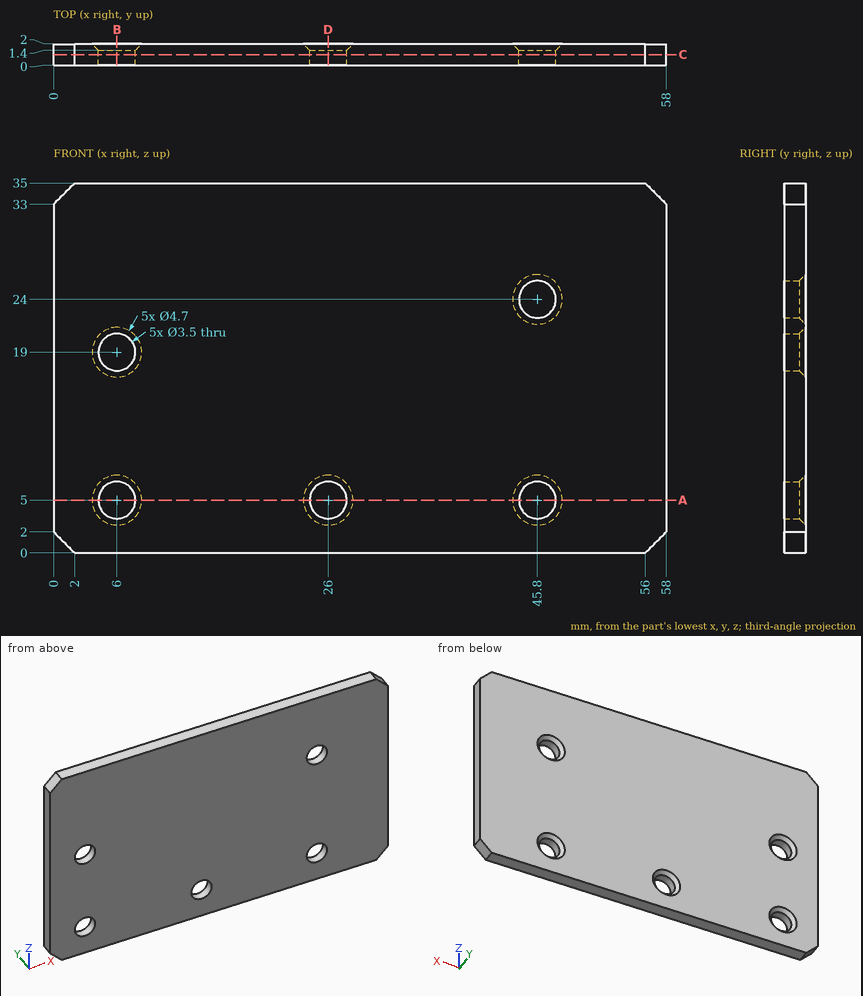
Drawing for the job (mm, zero at the part's lowest x, y, z). Give positions to 0.01 mm unless a question says otherwise; leave off trailing zeros. Order: outer loops, then holes, each group sorted by start corner. A loop starts at its lowest first (then second) coordinate and runs counter-clockwise, first axis right, second up. Notation, with made-up numbers: M -2,6 L 57,6 A29 cw 57,42 Z; hole C 80,-6.5 d5. An arc over 180 degrees is marked long. Use a Markdown table: item, result. Add a question column.
(1) Saw through at D-D, the plane x = 26. Give the cut face in (y, z).
(2) Drop flat-ended pins along their axis: P1, Ø4.5, axis at x = 6, z = 19, coming from the +Y side; P2, Ø5, axis at x = 26, z = 5, coming from the +Y side; P3, Ø3, axis at x = 45.8, z = 5, coming from the +Y side. Give the stop position or say it passes through.
(3) Probe line 1 along Z through (x, y) = (6, 1.1); line 2 along X through (y, z) = (1.1, 5); line 3 along X through (y, z) = (1.05, 24). List the from-to ranges inside material, lowest first. Write a range as [from, to].
(4) Saw through at B-B, the plane x = 6. Give the cut face in (y, z), and give its area (3 significant figures).
(5) Saw through at A-A, the plane z = 5. Give the cut face in (x, y), and give its area (3 significant figures).
(6) Saw through at C-C, the plane y = 1. Give the cut face in (x, z), and give its area (3 significant figures).
Answer key:
| question | item | result |
|---|---|---|
| 1 | outline | M 0,0 L 2,0 L 2,2.65 L 1.4,3.25 L 0,3.25 Z; M 0,6.75 L 1.4,6.75 L 2,7.35 L 2,35 L 0,35 Z |
| 2 | P1 | y = 1.9 |
| 2 | P2 | y = 2 |
| 2 | P3 | through |
| 3 | line 1 | [0, 3.25], [6.75, 17.25], [20.75, 35] |
| 3 | line 2 | [0, 4.25], [7.75, 24.25], [27.75, 44.05], [47.55, 58] |
| 3 | line 3 | [0, 44.05], [47.55, 58] |
| 4 | outline | M 0,0 L 2,0 L 2,2.65 L 1.4,3.25 L 0,3.25 Z; M 0,6.75 L 1.4,6.75 L 2,7.35 L 2,16.65 L 1.4,17.25 L 0,17.25 Z; M 0,20.75 L 1.4,20.75 L 2,21.35 L 2,35 L 0,35 Z |
| 4 | area | 55.3 mm^2 |
| 5 | outline | M 0,0 L 4.25,0 L 4.25,1.4 L 3.65,2 L 0,2 Z; M 7.75,0 L 24.25,0 L 24.25,1.4 L 23.65,2 L 8.35,2 L 7.75,1.4 Z; M 27.75,0 L 44.05,0 L 44.05,1.4 L 43.45,2 L 28.35,2 L 27.75,1.4 Z; M 47.55,0 L 58,0 L 58,2 L 48.15,2 L 47.55,1.4 Z |
| 5 | area | 93.9 mm^2 |
| 6 | outline | M 0,2 L 2,0 L 56,0 L 58,2 L 58,33 L 56,35 L 2,35 L 0,33 Z; hole C 6,5 d3.5; hole C 6,19 d3.5; hole C 26,5 d3.5; hole C 45.8,5 d3.5; hole C 45.8,24 d3.5 |
| 6 | area | 1,970 mm^2 |
